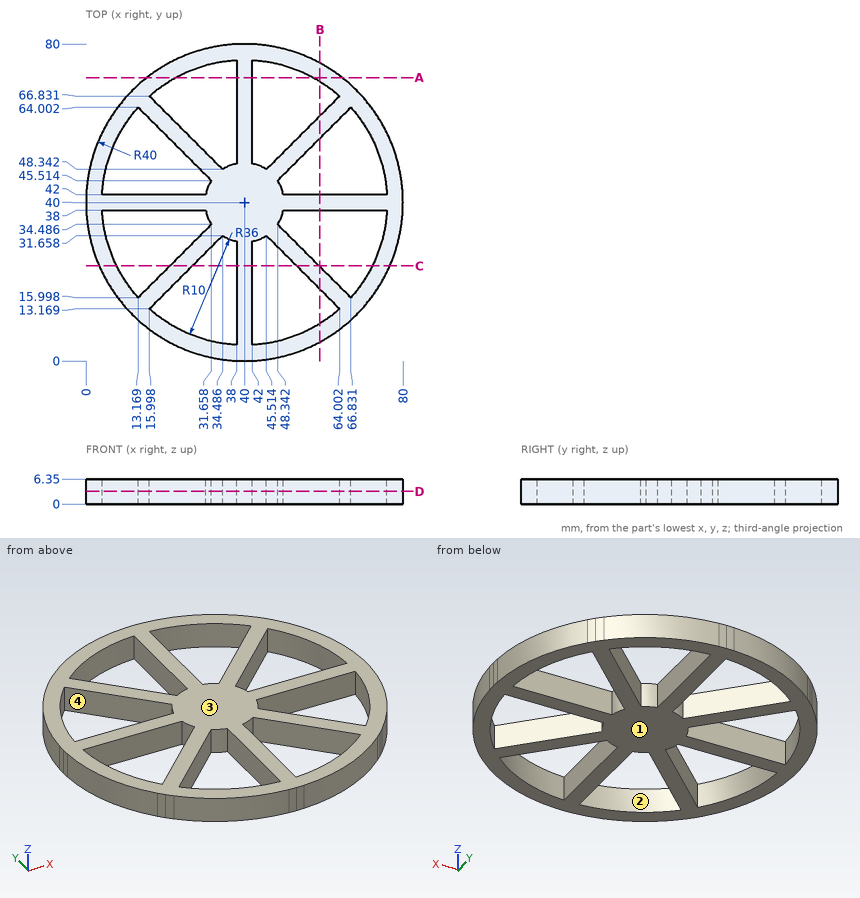
Could you check a few things on this drawing? It's one solid part, dimensions in mm from its lowest x, y, z. A direction names the side the tool comes from. Round coordinates to 2 decimals unless told otherwise and drop trailing zeros. Order: outer loops, then holes, each group sorted by start corner. A loop starts at its lowest first (then second) coordinate and runs counter-clockwise, first axis right, second up. Notation, with made-up numbers: M 5,-14 L 30,-14 A24 cw 30,24 Z; hole C 66,-21 d11. An arc over 180 degrees is marked long. One line per item, written item: value.
(1) Imagine slicing it at A-A (y = 71.5). Write out the boundary of the cut face in (x, z).
Ans:
outline: M 15.35,0 L 22.57,0 L 22.57,6.35 L 15.35,6.35 Z; M 38,0 L 42,0 L 42,6.35 L 38,6.35 Z; M 57.43,0 L 64.65,0 L 64.65,6.35 L 57.43,6.35 Z
(2) Which directions (+Z, -Z, +X, -X, +Y, -Y) give clear straight access to the entire face, cutting with the end or side of a thin tool? Please do the marked faces 3 and 4.
Ans:
face 3: +Z, +X, -X, +Y, -Y
face 4: +Z, -Z
(3) I'm going to push flat-ended pins straight in: P1, Ø8, axis at x = 69.5, y = 21.5, coming from the +Z side; P2, Ø1.9, axis at y = 22.5, z = 4, coming from the +X side (1 decimal); P3, Ø2, axis at y = 26.5, z = 3.5, coming from the +X side; P4, Ø1, axis at x = 21, z = 4.5, coming from the -Y side (1 decimal). Where does each tip first touch, or does it pass through?
Ans:
P1: stops at z = 6.35
P2: stops at x = 76.4
P3: stops at x = 78
P4: stops at y = 4.5
(4) Imagine slicing it at B-B (x = 59). Write out the boundary of the cut face in (y, z).
Ans:
outline: M 4.8,0 L 9.42,0 L 9.42,6.35 L 4.8,6.35 Z; M 18.17,0 L 23.83,0 L 23.83,6.35 L 18.17,6.35 Z; M 38,0 L 42,0 L 42,6.35 L 38,6.35 Z; M 56.17,0 L 61.83,0 L 61.83,6.35 L 56.17,6.35 Z; M 70.58,0 L 75.2,0 L 75.2,6.35 L 70.58,6.35 Z
(5) I need wall thicknesses on line 1 along Y through (x, z) = (45.5, 2.75); line 2 along X through (y, z) = (46.5, 4.25); line 3 along Y through (x, z) = (22, 0.5) (1 decimal). Which ranges of each line are inside material? Lowest first, please. Write a range as from..to.
Ans:
line 1: y = 0.38..4.42, 31.65..48.35, 75.58..79.62
line 2: x = 0.53..4.59, 30.67..49.33, 75.41..79.47
line 3: y = 4.3..8.8, 19.2..24.8, 38..42, 55.2..60.8, 71.2..75.7
(6) Imagine slicing it at C-C (y = 24). Write out the boundary of the cut face in (x, z), and give its area (3 significant figures).
Ans:
outline: M 3.34,0 L 7.75,0 L 7.75,6.35 L 3.34,6.35 Z; M 21.17,0 L 26.83,0 L 26.83,6.35 L 21.17,6.35 Z; M 38,0 L 42,0 L 42,6.35 L 38,6.35 Z; M 53.17,0 L 58.83,0 L 58.83,6.35 L 53.17,6.35 Z; M 72.25,0 L 76.66,0 L 76.66,6.35 L 72.25,6.35 Z
area: 153 mm^2
(7) If we mould it in two halves opening along X, with no side actions, what happens to the marked faces 1 and 2? For each: released by +X, released by -X, zero draft, split by the parting line, or undercut.
Ans:
face 1: zero draft
face 2: undercut
(8) Imagine slicing it at D-D (z = 3.25). Count the separate pieces of the cut face and the enclosed holes in it, and give its area (3 significant figures).
Ans:
separate pieces: 1
enclosed holes: 8
area: 2,100 mm^2
